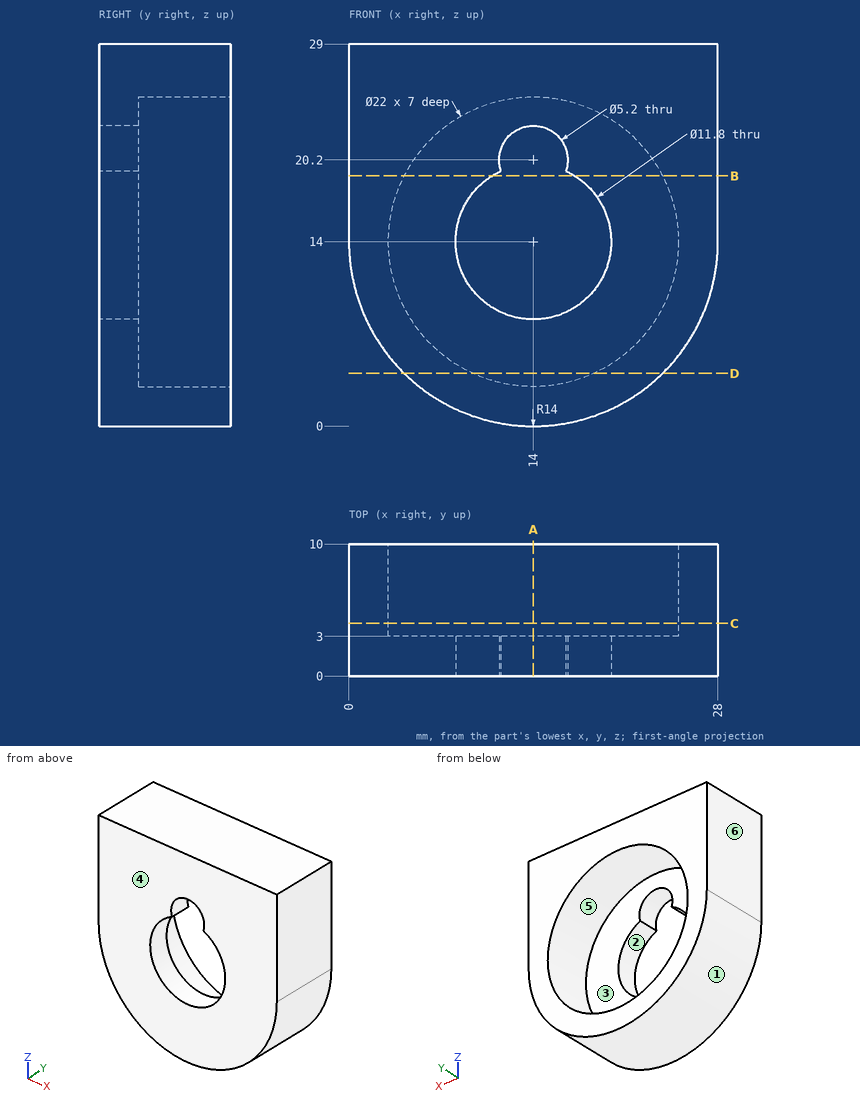
Design review of the part shown in the three views and the two pictorial views. Dimensions are in mm from the part's minimum x, y and z. A direction names the side the tool comes from. Round coordinates to 2 decimals unless told otherwise and drop trailing zeros. Order: outer loops, then holes, each group sorted by start corner. A loop starts at its lowest first (then second) coordinate and runs counter-clockwise, first axis right, second up. Notation, with made-up numbers: (70, 31.5) - (118, 31.5) arc R34 cw to (118, 66.5) - close; hole circle Ø9 at (28, 19.5). An arc over 180 degrees is marked (long way). Answer in a Markdown table with one row per item.
(1) Mouldability with a two-part tool opening along Z and no side actions: class the marked faces 1, 2, 3 and 4 as released by +Z, released by -Z, zero draft, split by the parting line, or undercut.
Result set:
| item | result |
|---|---|
| face 1 | released by -Z |
| face 2 | undercut |
| face 3 | undercut |
| face 4 | zero draft |
(2) Clearance check with flat-ended pins moving along their axes: P1, Ø2, axis at y = 3, z = 3.5, coming from the +X side; P2, Ø1, axis at y = 6.5, z = 3, coming from the -X side; P3, Ø3, axis at x = 7.5, y = 2, coming from the -Z side; P4, Ø7, axis at x = 14, z = 14, coming from the -Y side. State where each tip first meets the part, or that it passes through.
Result set:
| item | result |
|---|---|
| P1 | stops at x = 24.28 |
| P2 | stops at x = 4.74 |
| P3 | stops at z = 0.92 |
| P4 | passes through |
(3) For line 1 (Z direction, x = 14, y = 2.1); line 2 (Z direction, x = 14, y = 3.75); line 3 (X direction, y = 0.75, z = 14), list the stretches that pass through material, from the lowest coordinate up. Write a range as from..to.
Result set:
| item | result |
|---|---|
| line 1 | z = 0..8.1, 22.8..29 |
| line 2 | z = 0..3, 25..29 |
| line 3 | x = 0..8.1, 19.9..28 |
(4) Take a section at C-C on y = 4. Write out the cut boundary in (x, z), plus the area to 3 significant figures.
Result set:
| item | result |
|---|---|
| outline | (0, 14) arc R14 ccw to (28, 14) - (28, 29) - (0, 29) - close; hole circle Ø22 at (14, 14) |
| area | 348 mm2 |
(5) Take a section at B-B on z = 19. Write out the cut boundary in (x, y), plus the area to 3 significant figures.
Result set:
| item | result |
|---|---|
| outline | (0, 0) - (10.87, 0) - (10.87, 3) - (4.2, 3) - (4.2, 10) - (0, 10) - close; (17.13, 0) - (28, 0) - (28, 10) - (23.8, 10) - (23.8, 3) - (17.13, 3) - close |
| area | 124 mm2 |
(6) Take a section at A-A on x = 14. Write out the cut boundary in (y, z).
Result set:
| item | result |
|---|---|
| outline | (0, 0) - (10, 0) - (10, 3) - (3, 3) - (3, 8.1) - (0, 8.1) - close; (0, 22.8) - (3, 22.8) - (3, 25) - (10, 25) - (10, 29) - (0, 29) - close |
(7) Take a section at D-D on z = 4. Write out the cut boundary in (x, y), plus the area to 3 significant figures.
Result set:
| item | result |
|---|---|
| outline | (4.2, 0) - (23.8, 0) - (23.8, 10) - (18.58, 10) - (18.58, 3) - (9.42, 3) - (9.42, 10) - (4.2, 10) - close |
| area | 132 mm2 |
(8) Machinability: for the marked faces 5 and 6, which of the approach directions +Z, -Z, +X, -X, +Y, -Y give a long, thin tool a straight path to every point of the face, cutting with its end or side? Answer none if there is none.
Result set:
| item | result |
|---|---|
| face 5 | +Y |
| face 6 | +Z, -Z, -X, +Y, -Y |
